Part model, mm, in its own coordinate system. Face numbers are marked on the shaded views. Round coordinates to 2 decimals unless told otherwise and drop trailing zeros. Loops run counter-clockwise (first coordinate to the right, second up) from the corner with the lowest first, then second, coordinate; pieces in that order, holes last. Notation, with made-up numbers: (75, -5.5) - (93, -5.5) arc R28 cw to (93, 22.5) - close; hole circle Ø2 at (-17, 77). An arc over 180 degrees is marked (long way). Write each question's results on one line, items separated by ' | '. Start each with the question number.
(1) Flat gauge pin, fed straight in: P1, Ø2, axis at y = 47.62, z = 20.09, coming from the -X side. Where does the tip first touch, or does it go through?
(2) Cut at A-A, the plane y = 21. List the corners of the cut face in (x, z).
(3) Drill centre lines: L1, parallel to Y at x = 4, z = 1.5; L2, parallel to Z at x = -5.25, y = 26; L3, parallel to Z at x = 4, y = 32.5. Where is each one in solid material? Low to high.
(4) Mould opens along Z. For the marked faces 1, 2 and 3 say: released by +Z, released by -Z, zero draft, split by the parting line, or undercut.
(5) Cut at D-D, the plane z = 17. List the corners of the cut face in (x, y), then the cut area to 3 significant figures.
(6) Cut at B-B, the plane z = -12. List the corners of the cut face in (x, y), then the cut area to 3 significant figures.
(7) Cut at C-C, the plane x = -0.5. Give the number of separate pieces and of enclosed holes in the cut face, then the cut area to 3 significant figures.
Autodesk Inventor part; units mm, degrees
ref_plane "YZ Plane" through (0, 0, 0) normal (1, 0, 0) x (0, 1, 0)
ref_plane "XZ Plane" through (0, 0, 0) normal (0, 1, 0) x (-1, 0, 0)
ref_plane "XY Plane" through (0, 0, 0) normal (0, 0, 1) x (1, 0, 0)
sketch "Sketch1" plane through (0, 0, 0) normal (0, 1, 0) x (-1, 0, 0)
  line L0 (7.4947, 23.2617) -> (-5.2053, 23.2617)
  line L1 (-5.2053, 23.2617) -> (-5.2053, -14.8383)
  line L2 (-5.2053, -14.8383) -> (7.4947, -14.8383)
  line L3 (7.4947, -14.8383) -> (7.4947, 23.2617)
  point P0 (0, 0)
  dimension "d0" = 38.1
  dimension "d1" = 12.7
extrude "Extrusion1" add sketch "Sketch1" along normal blind 50.8
sketch "Sketch2" plane through (5.2053, 0, 23.2617) normal (1, 0, 0) x (0, 0, -1)
  line L0 (13.4782, 31.6) -> (24.9782, 31.6)
  line L1 (24.9782, 31.6) -> (24.9782, 38.1)
  line L2 (24.9782, 38.1) -> (13.4782, 38.1)
  line L3 (13.4782, 38.1) -> (13.4782, 31.6)
  line L4 (13.4782, 18.9) -> (24.9782, 18.9)
  line L5 (24.9782, 18.9) -> (24.9782, 25.4)
  line L6 (24.9782, 25.4) -> (13.4782, 25.4)
  line L7 (13.4782, 25.4) -> (13.4782, 18.9)
  line L8 (0, 0) -> (0, 50.8)
  line L9 (0, 0) -> (38.1, 0)
  line L10 (19.05, 56.7236) -> (19.05, -6.6913)
  point P0 (23.2617, 0)
  dimension "d4" = 11.5
  dimension "d5" = 0
  dimension "d6" = 0
  dimension "d8" = 25.4
  dimension "d9" = 12.7
  dimension "d10" = 6.5
  dimension "d11" = 6.5
  dimension "d47" = 19.05
extrude "Extrusion2" cut sketch "Sketch2" against normal blind 1.524
sketch "Sketch3" plane through (3.6813, 0, 23.2617) normal (1, 0, 0) x (0, 0, -1)
  circle A0 centre (21.8032, 22.225) radius 1.75
  circle A1 centre (16.6532, 22.225) radius 1.75
  line L0 (13.4782, 25.4) -> (24.9782, 25.4)
  line L1 (13.4782, 18.9) -> (13.4782, 25.4)
  line L2 (24.9782, 25.4) -> (24.9782, 18.9)
  circle A2 centre (16.6532, 34.925) radius 1.75
  circle A3 centre (21.8032, 34.9504) radius 1.75
  line L3 (13.4782, 38.1) -> (24.9782, 38.1)
  point P0 (23.2617, 0)
  dimension "d15" = 3.5
  dimension "d16" = 3.5
  dimension "d17" = 3.175
  dimension "d18" = 3.175
  dimension "d19" = 3.175
  dimension "d20" = 3.175
  dimension "d21" = 3.5
  dimension "d22" = 3.5
  dimension "d23" = 3.175
  dimension "d24" = 3.1496
  dimension "d48" = 0
  dimension "d49" = 0
extrude "Extrusion3" cut sketch "Sketch3" against normal blind 41.3385
sketch "Sketch4" plane through (0, 0, 0) normal (0, -1, 0) x (1, 0, 0)
  line L0 (5.2053, -14.8383) -> (-7.4947, -14.8383)
  line L1 (5.2053, 23.2617) -> (5.2053, -14.8383)
  point P0 (0, 0)
  point P1 (-1.1447, 16.9117)
  point P2 (-1.1447, -8.4883)
  dimension "d27" = 25.4
  dimension "d28" = 6.35
  dimension "d29" = 6.35
  dimension "d30" = 0
hole "Hole1" at (-1.1447, 0, 16.9117) at (-1.1447, 0, -8.4883) direction (0, 1, 0) diameter 3.683 end through all
sketch "Sketch5" plane through (0, 0, 0) normal (0, -1, 0) x (1, 0, 0)
  arc A0 (-5.3775, 4.7968) -> (-5.4627, 13.2795) centre (-5.4627, 9.0377) ccw
  arc A1 (-5.4627, -4.8561) -> (-5.4627, 3.6275) centre (-5.4627, -0.6143) ccw
  line L0 (-7.4947, -14.8383) -> (-7.4947, 23.2617)
  line L1 (-7.4947, 23.2617) -> (5.2053, 23.2617)
  line L2 (5.2053, -14.8383) -> (-7.4947, -14.8383)
  line L3 (-7.4947, -4.8561) -> (-5.4627, -4.8561)
  line L4 (-7.4947, 3.6275) -> (-5.4627, 3.6275)
  line L5 (-7.4947, 4.7542) -> (-5.3775, 4.7968)
  line L6 (-7.4947, 13.2795) -> (-5.4627, 13.2795)
  point P0 (0, 0)
  dimension "d38" = 8.4836
  dimension "d39" = 8.4836
  dimension "d42" = 14.224
  dimension "d43" = 14.224
  dimension "d50" = 0
  dimension "d51" = 2.032
  dimension "d67" = 4.2418
  dimension "d68" = 4.2418
  dimension "d69" = 4.2418
  dimension "d70" = 4.2418
extrude "Extrusion4" cut sketch "Sketch5" against normal blind 76.2
sketch "Sketch7" plane through (-7.4947, 0, 23.2617) normal (-1, 0, 0) x (0, 0, 1)
  line L0 (-38.1, 0) -> (-38.1, 50.8)
  line L1 (-38.1, 0) -> (-28.1178, 0)
  line L2 (-38.1, 50.8) -> (-28.1178, 50.8)
  line L3 (0, 0) -> (0, 50.8)
  point P0 (-23.2617, 0)
  point P1 (-34.925, 3.175)
  point P2 (-34.925, 47.625)
  point P3 (-27.821, 0)
  point P4 (-27.821, 50.8)
  point P5 (-3.175, 3.175)
  point P6 (-3.175, 47.625)
  dimension "d52" = 0
  dimension "d53" = 3.175
  dimension "d54" = 3.175
  dimension "d55" = 3.175
  dimension "d56" = 0
  dimension "d57" = 3.175
  dimension "d58" = 0
  dimension "d59" = 0
hole "Hole2" at (-7.4947, 3.175, -11.6633) at (-7.4947, 47.625, -11.6633) at (-7.4947, 3.175, 20.0867) at (-7.4947, 47.625, 20.0867) direction (1, 0, 0) diameter 2.4638 end through all
properties part number "PowerPlugBlock"
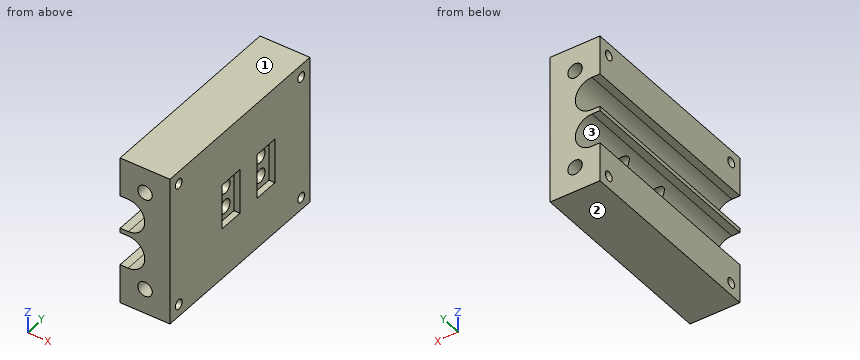
A:
1) P1: through
2) outline: (-7.49, -14.84) - (5.21, -14.84) - (5.21, -1.72) - (3.68, -1.72) - (3.68, 0.21) - (-1.3, 0.21) arc R4.24 cw to (-5.46, -4.86) - (-7.49, -4.86) - close; (-7.49, 3.63) - (-5.46, 3.63) arc R4.24 cw to (-2.83, 2.71) - (3.68, 2.71) - (3.68, 5.36) - (-3.35, 5.36) arc R4.24 cw to (-5.38, 4.8) - (-7.49, 4.75) - close; (-7.49, 13.28) - (-5.46, 13.28) arc R4.24 cw to (-1.39, 7.86) - (3.68, 7.86) - (3.68, 9.78) - (5.21, 9.78) - (5.21, 23.26) - (-7.49, 23.26) - close; hole circle Ø3.68 at (-1.14, -8.49); hole circle Ø3.68 at (-1.14, 16.91)
3) L1: 0 to 18.9, 25.4 to 31.6, 38.1 to 50.8 | L2: -14.84 to -4.85, 3.62 to 4.8, 13.27 to 23.26 | L3: -14.84 to -1.72, 9.78 to 23.26
4) face 1: released by +Z | face 2: released by -Z | face 3: undercut
5) outline: (-7.49, 0) - (-2.98, 0) - (-2.98, 50.8) - (-7.49, 50.8) - close; (0.69, 0) - (5.21, 0) - (5.21, 50.8) - (0.69, 50.8) - close | area: 458 mm2
6) outline: (-7.49, 0) - (5.21, 0) - (5.21, 1.99) - (-7.49, 1.99) - close; (-7.49, 4.36) - (5.21, 4.36) - (5.21, 46.44) - (-7.49, 46.44) - close; (-7.49, 48.81) - (5.21, 48.81) - (5.21, 50.8) - (-7.49, 50.8) - close | area: 585 mm2
7) separate pieces: 3 | enclosed holes: 8 | area: 1,530 mm2
